Input: part model. Units: mm. Frame: model coordinates. Face numbers are marked on the shaded views. A direction names the side the tool comes from. Coordinates: 2 decimals unless noted, no trailing zeros. Order: outer loops, then holes, each group sorted by start corner. A loop starts at its lowest first (then second) coordinate and runs counter-clockwise, first axis right, second up. Notation, with made-up numbers: (27.5, -32.5) - (61.5, -32.5) arc R11 cw to (61.5, -18.5) - close; hole circle Ø8 at (69, 14). An arc over 180 degrees is marked (long way). One line per question, with ' | ' between items.
Autodesk Inventor part; units mm, degrees
ref_plane "YZ Plane" through (0, 0, 0) normal (1, 0, 0) x (0, 1, 0)
ref_plane "XZ Plane" through (0, 0, 0) normal (0, 1, 0) x (-1, 0, 0)
ref_plane "XY Plane" through (0, 0, 0) normal (0, 0, 1) x (1, 0, 0)
sketch "Sketch1" plane through (0, 0, 0) normal (1, 0, 0) x (0, 1, 0)
  circle A0 centre (0, 0) radius 10
  circle A1 centre (0, 0) radius 14
  dimension "d0" = 20
  dimension "d1" = 28
extrude "Extrusion1" add sketch "Sketch1" along normal blind 15
sketch "Sketch2" plane through (15, 0, 0) normal (1, 0, 0) x (0, 0, -1)
  point P0 (0, 0)
sketch "Sketch3" plane through (15, 0, 0) normal (1, 0, 0) x (0, 0, -1)
  circle A0 centre (0, 0) radius 10
  line L0 (-12, 0) -> (-12, 12)
  line L1 (-12, 12) -> (46, 12)
  line L2 (46, 12) -> (46, -12)
  line L3 (46, -12) -> (-12, -12)
  line L4 (-12, -12) -> (-12, 0)
  line L5 (-15, 0) -> (-15, -12)
  line L6 (-15, 0) -> (-15, 12)
  line L7 (-12, 15) -> (46, 15)
  line L8 (49, 12) -> (49, -12)
  line L9 (46, -15) -> (-12, -15)
  arc A1 (49, 12) -> (46, 15) centre (46, 12) ccw
  arc A2 (46, -15) -> (49, -12) centre (46, -12) ccw
  arc A3 (-15, -12) -> (-12, -15) centre (-12, -12) ccw
  arc A4 (-12, 15) -> (-15, 12) centre (-12, 12) ccw
extrude "Extrusion2" add sketch "Sketch3" along normal blind 33 contours L6 A4 L7 A1 L8 A2 L9 A3 L5
sketch "Sketch4" plane through (15, 0, 0) normal (1, 0, 0) x (0, 0, -1)
  line L0 (-12, -12) -> (-12, 12)
  line L1 (7.2111, 12) -> (46, 12)
  line L2 (-12, 12) -> (46, 12)
  line L3 (46, 12) -> (46, -12)
  line L4 (46, -12) -> (-12, -12)
  line L5 (46, -12) -> (-12, -12)
  line L6 (-12, 12) -> (46, 12)
  line L7 (-12, -12) -> (-12, 12)
  point P0 (0, 0)
extrude "Extrusion3" add sketch "Sketch4" along normal blind 3
sketch "Sketch5" plane through (15, 0, 0) normal (-1, 0, 0) x (0, 0, 1)
  circle A0 centre (0, 0) radius 10
extrude "Extrusion4" cut sketch "Sketch5" against normal blind 3
sketch "Sketch6" plane through (15, -12, -49) normal (0, 0, -1) x (-1, 0, 0)
  point P0 (15, 12)
sketch "Sketch7" plane through (15, -12, -49) normal (0, 0, -1) x (-1, 0, 0)
  line L0 (0, 0) -> (0, -3)
  line L1 (0, -3) -> (0, 27)
  point P0 (15, 12)
  dimension "d22" = 30
sketch "Sketch8" plane through (15, -12, -49) normal (0, 0, -1) x (-1, 0, 0)
  point P0 (0, -3)
  point P1 (-3, 0)
sketch "Sketch9" plane through (15, -12, -49) normal (0, 0, -1) x (-1, 0, 0)
  line L0 (0, 27) -> (0, 24)
  line L1 (0, 27) -> (-64, 27)
  line L2 (-64, 27) -> (-64, -3)
  line L3 (0, -3) -> (-33, -3)
  line L4 (-64, -3) -> (0, -3)
  line L5 (0, -3) -> (0, 27)
  line L6 (0, 0) -> (0, 24)
  line L7 (-3, 24) -> (-3, 0)
  line L8 (-3, 0) -> (-3, 24)
  line L9 (0, 24) -> (-33, 24)
  line L10 (-3, 24) -> (-61, 24)
  line L11 (-61, 24) -> (-61, 0)
  line L12 (-61, 0) -> (-3, 0)
  line L13 (0, 0) -> (-33, 0)
  point P0 (15, 12)
  dimension "d27" = 64
  dimension "d28" = 30
  dimension "d29" = 58
extrude "Extrusion5" add sketch "Sketch9" along normal blind 30 contours L0 L9 L10 L11 L12 L13 L5 L3 L4 L2 L1 | L5 L13 L7 L9
sketch "Sketch10" plane through (48, 12, -49) normal (0, 0, -1) x (-1, 0, 0)
  line L0 (33, 3) -> (-31, 3)
  line L1 (33, 3) -> (33, 0)
  line L2 (-31, 3) -> (33, 3)
  line L3 (33, 3) -> (33, -27)
  line L4 (33, 0) -> (33, -24)
  line L5 (-31, 3) -> (-31, -27)
  line L6 (33, -27) -> (-31, -27)
  line L7 (-31, -27) -> (-31, 3)
  point P0 (48, -12)
  dimension "d32" = 30
extrude "Extrusion6" add sketch "Sketch10" against normal blind 5
fillet "Fillet1" radius 3 2 edges at (79, 15, -61.5) (79, -15, -61.5)
sketch "Sketch11" plane through (48, 12, -44) normal (0, 0, 1) x (1, 0, 0)
  line L0 (31, -24) -> (31, 0)
  line L1 (31, -12) -> (29, -12)
  line L2 (29, -12) -> (19, -12)
  circle A0 centre (19, -12) radius 10
  point P0 (-48, -12)
  dimension "d36" = 2
  dimension "d37" = 10
extrude "Extrusion7" cut sketch "Sketch11" against normal blind 10.5
sketch "Sketch12" plane through (48, 12, -44) normal (0, 0, 1) x (1, 0, 0)
  arc A0 (28, -7.6411) -> (28, -16.3589) centre (19, -12) ccw
  circle A1 centre (19, -12) radius 10
  circle A2 centre (19, -12) radius 10
  circle A3 centre (19, -12) radius 14
  point P0 (-48, -12)
  point P1 (28, -16.3589)
  dimension "d40" = 28
extrude "Extrusion8" add sketch "Sketch12" along normal blind 15
sketch "Sketch13" plane through (15, -12, 15) normal (0, 0, 1) x (1, 0, 0)
  line L0 (33, 0) -> (3, 0)
  line L1 (0, -3) -> (33, -3)
  line L2 (30.6116, 0) -> (33.6116, 0) construction
  line L3 (33, 0) -> (33, 24)
  line L4 (33, 3) -> (23, 3)
  line L5 (23, 3) -> (23, 20.8588)
  line L6 (23, 20.8588) -> (33, 20.8588)
  point P0 (-15, 12)
extrude "Extrusion9" cut sketch "Sketch13" against normal blind 21.75
sketch "Sketch14" plane through (79, -12, -79) normal (1, 0, 0) x (0, 0, -1)
  line L0 (-35, 24) -> (0, 24)
  line L1 (-3.7826, 24) -> (-0.7826, 24) construction
  line L2 (0, 0) -> (-35, 0)
  line L3 (-3.2489, 0) -> (-0.2489, 0) construction
  line L4 (0, 24) -> (0, 0)
  line L5 (0, 3) -> (-10, 3)
  line L6 (0, 3) -> (10, 3) construction
  line L7 (-10, 3) -> (-10, 21)
  line L8 (-10, 21) -> (0, 21)
  point P0 (-79, 12)
  dimension "d53" = 10
  dimension "d54" = 180
extrude "Extrusion10" cut sketch "Sketch14" against normal blind 25.75
sketch "Sketch15" plane through (15, -12, -79) normal (0, 0, -1) x (-1, 0, 0)
  line L0 (8.5716, 47.3564) -> (-2.6139, -49.713)
  line L1 (-2.6139, -49.713) -> (-66.1269, -32.0991)
  line L2 (-66.1269, -32.0991) -> (-83.6498, 8.8041)
  line L3 (-83.6498, 8.8041) -> (-71.64, 52.1092)
  line L4 (-71.64, 52.1092) -> (-17.9136, 47.3564)
  arc A0 (-17.9136, 47.3564) -> (-17.9136, 47.3564) centre (-16.407, 64.3867) ccw
  line L5 (-17.9136, 47.3564) -> (8.5716, 47.3564)
  point P0 (15, 12)
extrude "Extrusion11" cut sketch "Sketch15" against normal blind 30 contours L0 L1 L2 L3 L4 A0 L5 | A0 L5 picked at (-16.2394, 47.3367)
sketch "Sketch16" plane through (15, 15, 12) normal (0, 1, 0) x (1, 0, 0)
  line L0 (33, 56) -> (33, 0)
  line L1 (33, 35.3995) -> (33, 94.1554)
  line L2 (33, 94.1554) -> (79.7551, 84.127)
  line L3 (79.7551, 84.127) -> (69.5982, 12)
  line L4 (69.5982, 12) -> (67.3209, 12.3207)
  line L5 (67.3209, 12.3207) -> (33, 35.3995)
  point P0 (-15, 12)
extrude "Extrusion12" cut sketch "Sketch16" against normal blind 77.25
sketch "Sketch18" plane through (48, -15, -49) normal (0, 0, -1) x (-1, 0, 0)
  point P0 (48, 15)
fillet "Fillet2" radius 3 2 edges at (31.5, 15, -49) (31.5, -15, -49)
sketch "Sketch19" plane through (48, -12, -49) normal (0, 0, -1) x (-1, 0, 0)
  line L0 (-10.3978, 34.6876) -> (55.1217, 36.4172)
  line L1 (55.1217, 36.4172) -> (42.8113, -19.5389)
  line L2 (42.8113, -19.5389) -> (-1.2413, -25.4397)
  arc A0 (-1.2413, -25.4397) -> (-3.1744, -22.4893) centre (-5.2865, -25.9815) ccw
  line L3 (-3.1744, -22.4893) -> (-13.3482, 5.1835)
  arc A1 (-13.3482, 5.1835) -> (-11.3134, 8.4392) centre (-14.4287, 8.1225) ccw
  line L4 (-11.3134, 8.4392) -> (-10.3978, 34.6876)
  point P0 (48, 12)
extrude "Extrusion13" cut sketch "Sketch19" against normal blind 5
sketch "Sketch20" plane through (48, -12, -44) normal (0, 0, -1) x (-1, 0, 0)
  line L0 (0, 27) -> (0, 24)
  line L1 (0, 27) -> (33, 27)
  line L2 (33, 0) -> (33, -3)
  line L3 (33, 27) -> (33, -3)
  line L4 (33, -3) -> (0, -3)
  line L5 (33, -3) -> (0, -3)
  line L6 (0, -3) -> (0, 27)
  point P0 (48, 12)
extrude "Extrusion14" add sketch "Sketch20" along normal blind 3
fillet "Fillet3" radius 3 2 edges at (31.5, 15, -47) (31.5, -15, -47)
fillet "Fillet4" radius 1.5 4 edges at (48, 8.8588, 13.5) (38, 8.8588, 13.5) (38, -9, 13.5) (48, -9, 13.5)
properties part number "servo holder 1"
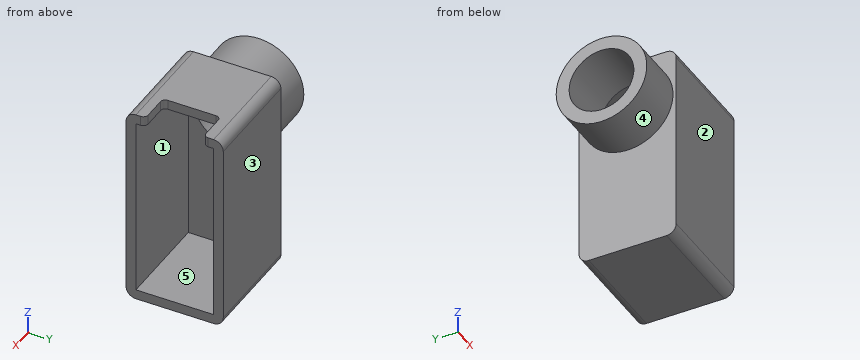
Item 1: Section B-B on y = -6.25. Return the cut outline in (x, z), and give its area (3 significant figures).
Data:
outline: (0, -12.53) - (15, -12.53) - (15, -47) - (48, -47) - (48, -44) - (18, -44) - (18, -7.81) - (0, -7.81) - close; (0, 7.81) - (18, 7.81) - (18, 12) - (38, 12) - (38, 15) - (15, 15) - (15, 12.53) - (0, 12.53) - close | area: 431 mm^2
Item 2: Contact query for flat-ended pins moving along their axis: P1, Ø10, axis at x = 13, y = 11, coming from the +Z side; P2, Ø1, axis at y = 8, z = -10, coming from the +X side; P3, Ø0.9, axis at x = 44, z = 13, coming from the -Y side; P4, Ø16, axis at y = 0, z = 0, coming from the -X side. Output: stop coordinate, or through.
Data:
P1: z = 15 | P2: x = 18 | P3: y = -14.95 | P4: through
Item 3: Section A-A on x = 26. Return the cut outline in (y, z), and give its area (3 significant figures).
Data:
outline: (-15, -44) arc R3 ccw to (-12, -47) - (12, -47) arc R3 ccw to (15, -44) - (15, 12) arc R3 ccw to (12, 15) - (-12, 15) arc R3 ccw to (-15, 12) - close; hole (-12, -44) - (12, -44) - (12, 12) - (-12, 12) - close | area: 508 mm^2
Item 4: Draft query along Z for the marked faces 3, 4 and 5. Return one class per face: released by +Z, released by -Z, zero draft, split by the parting line, or undercut.
Data:
face 3: zero draft | face 4: split by the parting line | face 5: undercut
Item 5: Ray query, line 1 (Z direction, x = 12, y = 0); line 2 (Y direction, x = 40, z = -41.5); line 3 (Z direction, x = 31.5, y = -11.25). Return the intervals inside material, ascending.
Data:
line 1: -14 to -10, 10 to 14 | line 2: -15 to -12, 12 to 15 | line 3: -47 to -44, 12 to 15
Item 6: Section D-D on y = -3. Return the cut outline in (x, z).
Data:
outline: (0, -13.67) - (15, -13.67) - (15, -47) - (48, -47) - (48, -44) - (18, -44) - (18, -9.54) - (0, -9.54) - close; (0, 9.54) - (18, 9.54) - (18, 12) - (38, 12) - (38, 15) - (15, 15) - (15, 13.67) - (0, 13.67) - close
Item 7: Access query for the marked faces 1 and 2. Directions: +Z, -Z, +X, -X, +Y, -Y. A direction counts if a zero-diameter tool reaches every point of the face in a straight line with its end or side. Return the directions, or none.
Data:
face 1: +X | face 2: +Z, -Z, +X, -X, -Y
Item 8: Section C-C on z = -22. Return the cut outline in (x, y), and give its area (3 significant figures).
Data:
outline: (15, -15) - (48, -15) - (48, -12) - (18, -12) - (18, 12) - (48, 12) - (48, 15) - (15, 15) - close | area: 270 mm^2
